Autodesk Inventor part; units mm, degrees
ref_plane "YZ Plane" through (0, 0, 0) normal (1, 0, 0) x (0, 1, 0)
ref_plane "XZ Plane" through (0, 0, 0) normal (0, 1, 0) x (-1, 0, 0)
ref_plane "XY Plane" through (0, 0, 0) normal (0, 0, 1) x (1, 0, 0)
sketch "스케치1" plane through (0, 0, 0) normal (0, 1, 0) x (-1, 0, 0)
  circle A0 centre (0, 0) radius 35
  circle A1 centre (0, 0) radius 7.5
  circle A2 centre (0, 0) radius 12.5
  circle A3 centre (0, 0) radius 30
  dimension "d0" = 70
  dimension "d1" = 15
  dimension "d2" = 25
  dimension "d3" = 60
extrude "돌출1" add sketch "스케치1" along normal blind 5
sketch "스케치2" plane through (0, 0, 0) normal (0, -1, 0) x (1, 0, 0)
  line L0 (-10.8253, 6.25) -> (-25.9808, 15)
  circle A0 centre (0, 0) radius 30
  circle A1 centre (0, 0) radius 7.5
  circle A2 centre (0, 0) radius 7.5
  circle A3 centre (0, 0) radius 12.5
  circle A4 centre (0, 0) radius 12.5
  line L1 (0, 12.5) -> (0, 30)
  line L2 (10.8253, 6.25) -> (25.9808, 15)
  line L3 (10.8253, -6.25) -> (25.9808, -15)
  line L4 (0, -12.5) -> (0, -30)
  line L5 (-10.8253, -6.25) -> (-25.9808, -15)
  line L6 (-1.5, 34.9678) -> (1.5, 34.9678)
  line L7 (1.5, 34.9678) -> (1.5, 12.4097)
  line L8 (1.5, 12.4097) -> (-1.5, 12.4097)
  line L9 (-1.5, 12.4097) -> (-1.5, 34.9678)
  circle A5 centre (0, 0) radius 35
  dimension "d10" = 3
  dimension "d11" = 1.5
extrude "돌출2" add sketch "스케치2" against normal blind 5 contours L9 A0 L1 A3 | L9 L6 L7 A0 | L1 A0 L7 A3
pattern_circular "원형 패턴1" count 6 over 360 about axis through (0, 0, 0) along (0, 1, 0) of "돌출2"
fillet "모깎기1" radius 1.9 2 edges at (35, 0, 0) (35, 5, 0)
sketch "스케치3" plane through (-26.6983, 0, -13.6822) normal (-0.5, 0, 0.866) x (0.866, 0, 0.5)
  line L0 (64.9625, 3.1) -> (-5.0375, 3.1)
  line L1 (-5.0375, 1.9) -> (64.9625, 1.9)
  point P0 (29.9625, 0)
  dimension "d18" = 1.2
ref_plane "작업 평면1" through (0, 2.5, 0) normal (0, 1, 0) x (1, 0, 0)
sketch "스케치4" plane through (0, 2.5, 0) normal (0, 1, 0) x (1, 0, 0)
  circle A0 centre (0, 0) radius 35
  circle A1 centre (0, 0) radius 34.4
  dimension "d19" = 0.6
extrude "돌출3" cut sketch "스케치4" along normal mid plane 1.2
sketch "스케치5" plane through (0, 5, 0) normal (0, 1, 0) x (1, 0, 0)
  point P0 (0, 0)
sketch "스케치6" plane through (0, 0, 0) normal (0, -1, 0) x (1, 0, 0)
  arc A0 (9.9971, 7.5039) -> (1.5, 12.4097) centre (0, 0) ccw
  circle A1 centre (0, 0) radius 12.5
  line L0 (-9.9971, 7.5039) -> (-25.1983, 16.2803)
  arc A2 (-1.5, 29.9625) -> (-25.1983, 16.2803) centre (0, 0) ccw
  line L1 (-1.5, 29.9625) -> (-1.5, 12.4097)
  arc A3 (-1.5, 12.4097) -> (-9.9971, 7.5039) centre (0, 0) ccw
  circle A4 centre (0, 0) radius 7.5
  arc A5 (9.9971, 7.5039) -> (1.5, 12.4097) centre (0, 0) ccw
  line L2 (1.5, 12.4097) -> (1.5, 29.9625)
  arc A6 (25.1983, 16.2803) -> (1.5, 29.9625) centre (0, 0) ccw
  line L3 (25.1983, 16.2803) -> (9.9971, 7.5039)
  arc A7 (11.4971, -4.9058) -> (11.4971, 4.9058) centre (0, 0) ccw
  line L4 (11.4971, 4.9058) -> (26.6983, 13.6822)
  arc A8 (26.6983, -13.6822) -> (26.6983, 13.6822) centre (0, 0) ccw
  line L5 (26.6983, -13.6822) -> (11.4971, -4.9058)
  arc A9 (1.5, -12.4097) -> (9.9971, -7.5039) centre (0, 0) ccw
  line L6 (9.9971, -7.5039) -> (25.1983, -16.2803)
  arc A10 (1.5, -29.9625) -> (25.1983, -16.2803) centre (0, 0) ccw
  line L7 (1.5, -29.9625) -> (1.5, -12.4097)
  arc A11 (-9.9971, -7.5039) -> (-1.5, -12.4097) centre (0, 0) ccw
  line L8 (-1.5, -12.4097) -> (-1.5, -29.9625)
  arc A12 (-25.1983, -16.2803) -> (-1.5, -29.9625) centre (0, 0) ccw
  line L9 (-25.1983, -16.2803) -> (-9.9971, -7.5039)
  arc A13 (-11.4971, 4.9058) -> (-11.4971, -4.9058) centre (0, 0) ccw
  line L10 (-11.4971, -4.9058) -> (-26.6983, -13.6822)
  arc A14 (-26.6983, 13.6822) -> (-26.6983, -13.6822) centre (0, 0) ccw
  line L11 (-26.6983, 13.6822) -> (-11.4971, 4.9058)
  circle A15 centre (0, 0) radius 33.1
  circle A16 centre (0, 0) radius 17.5
  dimension "d22" = 35
extrude "돌출4" add sketch "스케치6" along normal blind 1 contours A1 A0 | L3 A16 L4 A1 | A0 L2 A16 L3 | A1 L1 A16 L2 | L4 A16 L5 A1 | A1 L0 A16 L1 | A1 L11 A16 L0 | L5 A16 L6 A1 | A1 L10 A16 L11 | L6 A16 L7 A1 | A1 L9 A16 L10 | L7 A16 L8 A1 | A1 L8 A16 L9
sketch "스케치7" plane through (0, -1, 0) normal (0, -1, 0) x (1, 0, 0)
  circle A0 centre (0, 0) radius 12.5
  circle A1 centre (0, 0) radius 7.5
  circle A2 centre (0, 0) radius 7.5
  circle A3 centre (0, 0) radius 17.5
  dimension "d25" = 25
extrude "돌출5" add sketch "스케치7" along normal blind 3 contours A0
sketch "스케치8" plane through (0, -4, 0) normal (0, -1, 0) x (1, 0, 0)
  circle A0 centre (0, 0) radius 17.5
  circle A1 centre (0, 0) radius 17.5
  circle A2 centre (0, 0) radius 7.5
  circle A3 centre (0, 0) radius 12.5
  dimension "d28" = 35
extrude "돌출6" add sketch "스케치8" against normal blind 1 contours A0
sketch "스케치9" plane through (0, -4, 0) normal (0, -1, 0) x (1, 0, 0)
  circle A0 centre (0, 0) radius 7.5
sketch "스케치10" plane through (0, -3, 0) normal (0, 1, 0) x (-1, 0, 0)
  point P0 (0, 0)
fillet "모깎기2" radius 0.8 2 edges at (-17.5, -3, 0) (-17.5, -1, 0)
properties part number "뒷바퀴"
For this review, take the finished solid that the model builds, in its own axes (mm). A direction names the side the tool comes from. Give positions to 0.01 mm unless a question says otherwise; leave off trailing zeros. Order: outer loops, then holes, each group sorted by start corner. A loop starts at its lowest first (then second) coordinate and runs counter-clockwise, first axis right, second up. Notation, with made-up numbers: (-20.75, 86) -> (20.25, 86) arc R28 ccw to (20.25, 121) -> close; hole circle Ø6 at (1.25, -39). An arc over 180 degrees is marked (long way). Write item = value, one per line.
1) We need section B-B, the plane z = 0. Count the separate pieces of the cut face and the enclosed holes in it, and give its area (3 significant figures).
Findings:
separate_pieces = 4
enclosed_holes = 0
area = 155 mm^2
2) Insertion check: pin 1 (2.5 mm diameter, centred on y = 2, z = 21, fed in from +X); pin 2 (3 mm diameter, centred on x = 7.5, z = 14, fed in from +Y); pin 3 (1 mm diameter, centred on x = -12, y = 1, fed in from -Z). Each pin has a flat end and moves straight along its axis. Give the tip position at first contact, or say it passes through.
Findings:
pin_1 = 28.89
pin_2 = 0
pin_3 = -32.92
3) Draft analysis for pull direction X (two halves, no side actions). For faces 4 (the face through (19.204, 2.465, 9.355)), 5 (the face through (23, 3.1, 26)), 6 (the face through (-34.367, 2.508, -1.513)), state which applies: pulls with the +X half, pulls with the -X half, needs draft (parallel to the pull), parting line crosses it, or undercut.
Findings:
face_4 = undercut
face_5 = needs draft
face_6 = parting line crosses it
4) We need section C-C, the plane y = -2. Give the boundary of the cut face in (x, z).
Findings:
outline = circle Ø25 at (0, 0); hole circle Ø15 at (0, 0)
5) To check wall thickness, follow L1, parallel to X at y = -2, z = 0.5; L2, parallel to Z at x = 0, y = -0.5; L3, parallel to X at y = 1, z = 9.5. State the ranges of each line that lie inside material, in increasing order. Write a range as from..to.
Findings:
L1 = -12.49..-7.48, 7.48..12.49
L2 = -17.44..-7.5, 7.5..17.44
L3 = -33.45..-28.46, -19.45..-13.45, -8.12..8.12, 13.45..19.45, 28.46..33.45
6) For faces 1 (the face through (15, 0, -10)), 2 (the face through (6.1, -3, -11.1)), 3 (the face through (6.31, 2.46, 10.79)), list the 3-axis set-ups (+Z, -Z, +X, -X, +Y, -Y) from which the entire face can be reached by the end or side of a thin tool; tool diameter is ignored.
Findings:
face_1 = -Y
face_2 = none
face_3 = +Y
